```python
from build123d import *

# Parameters (mm, degrees)
SKETCH1_W           = 100
SKETCH1_H           = 50
BOSS_EXTRUDE1_DEPTH = 50
FILLET1_R           = 10
FILLET2_R           = 10


with BuildPart() as part:
    # Sketch1 → Boss-Extrude1 (new body)
    with BuildSketch(Plane(origin=(0, 0, 0), x_dir=(1, 0, 0), z_dir=(0, 1, 0))):
        Rectangle(SKETCH1_W, SKETCH1_H)
    extrude(amount=BOSS_EXTRUDE1_DEPTH)

    # Fillet1
    fillet1_edges = [part.edges().sort_by_distance(p)[0] for p in [
        (50, 50, 0),
        (0, 50, -25),
        (-50, 50, 0),
        (50, 0, 0),
        (0, 0, 25),
        (50, 25, -25),
        (50, 25, 25),
        (-50, 25, 25),
        (0, 50, 25),
    ]]
    fillet(fillet1_edges, radius=FILLET1_R)

    # Fillet2
    # the kernel refuses this fillet: 10 mm, written as the material it takes off along each edge
    with BuildSketch(Plane(origin=(-40, 10, 15), x_dir=(0, -1, 0), z_dir=(-1, 0, 0))) as fillet2_piece_1_section:
        Polygon((0, 0), (FILLET2_R, 0), (FILLET2_R, FILLET2_R), (0, FILLET2_R), align=None)
    fillet2_piece_1 = extrude(amount=FILLET2_R, mode=Mode.PRIVATE)
    fillet2_piece_1 = fillet2_piece_1 - Plane(origin=(-40, 10, 15), x_dir=(0, 0.7071067811865475, -0.7071067811865475), z_dir=(-1, 0, 0)) * Sphere(FILLET2_R, mode=Mode.PRIVATE)
    add(fillet2_piece_1, mode=Mode.SUBTRACT)
    with BuildSketch(Plane(origin=(-40, 40, -15), x_dir=(-1, 0, 0), z_dir=(0, 0, -1))) as fillet2_piece_2_section:
        Polygon((0, 0), (FILLET2_R, 0), (FILLET2_R, FILLET2_R), (0, FILLET2_R), align=None)
    fillet2_piece_2 = extrude(amount=FILLET2_R, mode=Mode.PRIVATE)
    fillet2_piece_2 = fillet2_piece_2 - Plane(origin=(-40, 40, -15), x_dir=(0.7071067811865475, -0.7071067811865475, 0), z_dir=(0, 0, -1)) * Sphere(FILLET2_R, mode=Mode.PRIVATE)
    add(fillet2_piece_2, mode=Mode.SUBTRACT)
    with BuildSketch(Plane(origin=(40, 10, -15), x_dir=(0, -1, 0), z_dir=(0, 0, -1))) as fillet2_piece_3_section:
        Polygon((0, 0), (FILLET2_R, 0), (FILLET2_R, -FILLET2_R), (0, -FILLET2_R), align=None)
    fillet2_piece_3 = extrude(amount=FILLET2_R, mode=Mode.PRIVATE)
    fillet2_piece_3 = fillet2_piece_3 - Plane(origin=(40, 10, -15), x_dir=(-0.7071067811865475, 0.7071067811865475, 0), z_dir=(0, 0, -1)) * Sphere(FILLET2_R, mode=Mode.PRIVATE)
    add(fillet2_piece_3, mode=Mode.SUBTRACT)
    with BuildSketch(Plane(origin=(-40, 10, -15), x_dir=(-1, 0, 0), z_dir=(0, 0, -1))) as fillet2_piece_4_section:
        Polygon((0, 0), (FILLET2_R, 0), (FILLET2_R, -FILLET2_R), (0, -FILLET2_R), align=None)
    fillet2_piece_4 = extrude(amount=FILLET2_R, mode=Mode.PRIVATE)
    fillet2_piece_4 = fillet2_piece_4 - Plane(origin=(-40, 10, -15), x_dir=(0.7071067811865475, 0.7071067811865475, 0), z_dir=(0, 0, -1)) * Sphere(FILLET2_R, mode=Mode.PRIVATE)
    add(fillet2_piece_4, mode=Mode.SUBTRACT)
    with BuildSketch(Plane(origin=(40, 0, -25), x_dir=(0, 1, 0), z_dir=(-1, 0, 0))) as fillet2_piece_5:
        with BuildLine():
            CenterArc((FILLET2_R, -FILLET2_R), FILLET2_R, 90, 90)
            Line((0, -FILLET2_R), (0, 0))
            Line((0, 0), (FILLET2_R, 0))
        make_face()
    extrude(amount=80, mode=Mode.SUBTRACT)
    with BuildSketch(Plane(origin=(-50, 10, -25), x_dir=(1, 0, 0), z_dir=(0, 1, 0)), Plane(origin=(-50, 0, -15), x_dir=(0, 1, 0), z_dir=(0, 0, 1))) as fillet2_piece_6:
        with BuildLine():
            CenterArc((FILLET2_R, -FILLET2_R), FILLET2_R, 90, 90)
            Line((0, -FILLET2_R), (0, 0))
            Line((0, 0), (FILLET2_R, 0))
        make_face()
    extrude(amount=30, mode=Mode.SUBTRACT)


solid = part.part
```
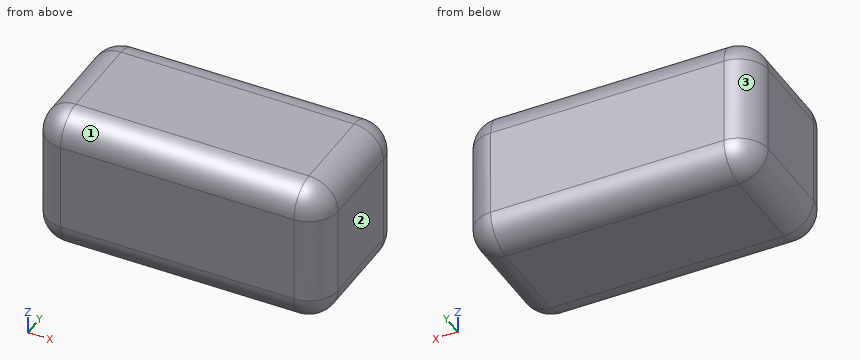
Model file for the job. Use its own axes, mm. Face numbers are marked on the shaded views. Coordinates: 2 decimals unless noted, no trailing zeros. Write each loop counter-clockwise with the first axis right and the second up, starting at its lowest first coordinate (ties: lowest second). Pieces come first, ordered by that corner, then holes. Notation, with made-up numbers: (28, 10.5) - (37, 10.5) arc R15 cw to (37, 34.5) - close; hole circle Ø2 at (-34, 70.5). An arc over 180 degrees is marked (long way). Use a Markdown table: item, result. Add a question column.
Item 1: Band-saw the part on A-A, the plane z = 2. Write the cut outline in (x, y), and give its area (3 significant figures).
Item 2: Drop flat-ended pins along their axis: pin 1 (5 mm diameter, centred on x = -12.5, y = 44, fed in from -Z); pin 2 (2 mm diameter, centred on y = 43, z = -1.5, fed in from +X). Give the stop position or say it passes through.
Item 3: Drill centre lines: line 1 along X through (y, z) = (9.5, 3.5); line 2 along Z through (x, y) = (42, 5.5); line 3 along X through (y, z) = (6, -7). Where is each one in solid material? Low to high.
Item 4: Two-plate mould, pull along X, no slides. Class the marked faces 1, 2 and 3: pulls with the +X half, pulls with the -X half, needs draft (parallel to the pull), parting line crosses it, or undercut.
Item 5: Band-saw the part on B-B, the plane y = 18.5. Write the cut outline in (x, z), and give its area (3 significant figures).
A:
| question | item | result |
|---|---|---|
| 1 | outline | (-50, 10) arc R10 ccw to (-40, 0) - (40, 0) arc R10 ccw to (50, 10) - (50, 40) arc R10 ccw to (40, 50) - (-40, 50) arc R10 ccw to (-50, 40) - close |
| 1 | area | 4,910 mm² |
| 2 | pin 1 | stops at z = -24.89 |
| 2 | pin 2 | stops at x = 49.8 |
| 3 | line 1 | x = -49.99 to 49.99 |
| 3 | line 2 | z = -23.7 to 23.7 |
| 3 | line 3 | x = -49.17 to 49.17 |
| 4 | face 1 | needs draft |
| 4 | face 2 | pulls with the +X half |
| 4 | face 3 | pulls with the -X half |
| 5 | outline | (-50, -15) arc R10 ccw to (-40, -25) - (40, -25) arc R10 ccw to (50, -15) - (50, 15) arc R10 ccw to (40, 25) - (-40, 25) arc R10 ccw to (-50, 15) - close |
| 5 | area | 4,910 mm² |
